```python
from build123d import *

# Parameters (mm, degrees)
SKETCH1_W          = 1400
SKETCH1_H          = 110
SKETCH3_W          = 241.229259038
SKETCH3_H          = 118.473208867
CUT_EXTRUDE1_DEPTH = 3000
SKETCH4_W          = 263.080499957
SKETCH4_H          = 130.335311081
CUT_EXTRUDE2_DEPTH = 1000


with BuildPart() as part:
    # Sweep2: sweep along a path in Sketch2
    with BuildLine(Plane(origin=(0, 0, 0), x_dir=(0, 0, -1), z_dir=(1, 0, 0))) as sweep2_path:
        Line((0, -52.72397822), (-373.826634648, -310.359400666))
    # Sketch1 → Sweep2 (sweep)
    with BuildSketch(Plane.XY):
        Rectangle(SKETCH1_W, SKETCH1_H)
    sweep(path=sweep2_path.line)

    # Sketch3 → Cut-Extrude1 (cut)
    with BuildSketch(Plane(origin=(0, 0, 0), x_dir=(0, 0, -1), z_dir=(1, 0, 0))):
        with Locations((-253.212005129, -261.87202688)):
            Rectangle(SKETCH3_W, SKETCH3_H)
    extrude(amount=CUT_EXTRUDE1_DEPTH, mode=Mode.SUBTRACT)

    # Sketch4 → Cut-Extrude2 (cut)
    with BuildSketch(Plane(origin=(0, 0, 0), x_dir=(0, 0, -1), z_dir=(1, 0, 0))):
        with Locations((-242.28638467, -267.803077986)):
            Rectangle(SKETCH4_W, SKETCH4_H)
    extrude(amount=-CUT_EXTRUDE2_DEPTH, mode=Mode.SUBTRACT)


solid = part.part
```
Here's how the part is built. I have some questions about the finished solid (model axes, mm). Round coordinates to 2 decimals unless told otherwise and drop trailing zeros. Loops run counter-clockwise (first coordinate to the right, second up) from the corner with the lowest first, then second, coordinate; pieces in that order, holes last. Notation, with made-up numbers: (53, 50.5) -> (107, 50.5) arc R32 ccw to (107, 76.5) -> close; hole circle Ø3 at (5.25, 14.25). An arc over 180 degrees is marked (long way). Answer as CSV lines item,"result". Start each with the question number.
1. Imagine slicing it at B-B on z = 73. Write out the boundary of the cut face in (x, y), plus the area to 3 significant figures.
2. Imagine slicing it at A-A on x = 516.5. Write out the boundary of the cut face in (y, z).
3. I'm going to push flat-ended pins straight in: P1, Ø1.5, axis at x = -56.5, z = 168.5, coming from the -Y side; P2, Ø4, axis at x = -272.5, y = -90, coming from the +Z side. Where does each tip first touch, or does it pass through?
4. I need wall thicknesses on probe 1 along Z at (x, y) = (-569.5, -98); probe 2 along Z at (x, y) = (115, -153); probe 3 along Y at (x, z) = (-221, 126). Which ranges of each line are inside material? Lowest first, please. Write a range as from..to.
Solution:
1,outline,"(-700, -105.31) -> (700, -105.31) -> (700, 4.69) -> (-700, 4.69) -> close"
1,area,"154,000 mm²"
2,outline,"(-202.64, 214.22) -> (-55, 0) -> (55, 0) -> (-202.64, 373.83) -> close"
3,P1,"y = -171.64"
3,P2,"z = 213.3"
4,probe 1,"62.39..222"
4,probe 2,"142.2..301.81"
4,probe 3,"-141.84..-31.84"
